```python
from build123d import *

# Parameters (mm, degrees)
IZIM1_W               = 153
IZIM1_H               = 12.405405405
KES_EKSTR_ZYON1_DEPTH = 21
KES_EKSTR_ZYON2_START = -21
KES_EKSTR_ZYON2_DEPTH = 21


with BuildPart() as part:
    # Çizim1 → Döndür1 (revolve)
    with BuildSketch(Plane(origin=(0, 0, 0), x_dir=(-1, 0, 0), z_dir=(0, 0, -1)), mode=Mode.PRIVATE) as d_nd_r1_sk:
        with Locations((-76.5, 6.202702703)):
            Rectangle(IZIM1_W, IZIM1_H)
    revolve(d_nd_r1_sk.sketch.rotate(Axis((153, 0, 0), (-1, 0, 0)), 270), axis=Axis((153, 0, 0), (-1, 0, 0)))

    # Çizim2 → Kes-Ekstrüzyon1 (cut)
    with BuildSketch(Plane(origin=(153, 0, 0), x_dir=(0, 0, -1), z_dir=(1, 0, 0))):
        with BuildLine():
            Line((5.478492651, -2.446654506), (11.327153725, -5.058623505))
            ThreePointArc((11.327153725, -5.058623505), (0.113988201, -12.404881699), (-11.232281693, -5.26592169))
            Line((-11.232281693, -5.26592169), (-5.432606832, -2.546916373))
            ThreePointArc((-5.432606832, -2.546916373), (-0.055131548, 5.999746704), (5.478492651, -2.446654506))
        make_face()
    extrude(amount=-KES_EKSTR_ZYON1_DEPTH, mode=Mode.SUBTRACT)

    # Çizim3 → Kes-Ekstrüzyon2 (cut)
    with BuildSketch(Plane.ZY.offset(KES_EKSTR_ZYON2_START)):
        with BuildLine():
            ThreePointArc((2.25, -5.562148865), (0, 6), (-2.25, -5.562148865))
            ThreePointArc((-2.25, -5.562148865), (0, -6), (2.25, -5.562148865))
        make_face()
    extrude(amount=KES_EKSTR_ZYON2_DEPTH, mode=Mode.SUBTRACT)


solid = part.part
```
Design review of the part built by this model. Coordinates are the model's own, in mm. A direction names the side the tool comes from. Give positions to 0.01 mm unless a question says otherwise; leave off trailing zeros. Order: outer loops, then holes, each group sorted by start corner. A loop starts at its lowest first (then second) coordinate and runs counter-clockwise, first axis right, second up. Notation, with made-up numbers: M -25.5,12.5 L 23.5,12.5 A24 ccw 23.5,44.5 Z; hole C 50,-28 d5. An arc over 180 degrees is marked long. One line per question, with ' | ' between items. Start each with the question number.
Q1. For L1, parallel to Z at x = 145.75, y = 0; L2, parallel to Y at x = 146, z = 0; L3, parallel to X at y = -2.75, z = 2, list the stretches that pass through material, from the lowest coordinate up. Write a range as [from, to].
Q2. We need section B-B (y = 0). Write out the cut boundary in (x, z), plus the area to 3 significant figures.
Q3. Machinability: for faces 1 (the face through (142.647, -3.925, 8.373)), 2 (the face through (143, 6, 0)), 3 (the face through (153, 6, -3)), 4 (the face through (21, 0, 0)), which of the approach directions +Z, -Z, +X, -X, +Y, -Y give a long, thin tool a straight path to every point of the face, cutting with its end or side? Answer none if there is none.
Q4. The part is to be moulded in two halves that separate along Z. For faces 5 (the face through (0, -3, 6)), 6 (the face through (75.4, 12.3, -1.6)), 7 (the face through (142.647, -3.734, -8.362)), say which applies: +Z half, -Z half, draft (parallel to the pull), parting line (faces both ways), or undercut.
Q5. For pin 1 Ø4 at (x, y) = (96, 7.5) entering from -Z; pin 2 Ø6 at (x, z) = (22.5, 8.5) entering from +Y; pin 3 Ø4 at (x, z) = (97, 5.5) entering from +Y; pin 4 Ø13 at (y, z) = (-3, 1) entering from -X, all flat-tipped, find the tip position at first contact; note any pin that passes through.
Q6. We need section D-D (x = 13). Write out the cut boundary in (y, z), plus the area to 3 significant figures.
Q7. We need section C-C (x = 37.5). Write out the cut boundary in (y, z), plus the area to 3 significant figures.
Q8. We need section A-A (z = 0). Write out the cut boundary in (x, y).
Returned:
1) L1: [-12.41, -6], [6, 12.41] | L2: [6, 12.41] | L3: [21, 132]
2) outline: M 0,-12.41 L 153,-12.41 L 153,-6 L 132,-6 L 132,6 L 153,6 L 153,12.41 L 0,12.41 L 0,6 L 21,6 L 21,-6 L 0,-6 Z | area: 3,290 mm2
3) face 1: +X, -Y | face 2: +X | face 3: +Z, -Z, +X, +Y, -Y | face 4: -X
4) face 5: draft | face 6: parting line | face 7: undercut
5) pin 1: z = -11.12 | pin 2: y = 11.12 | pin 3: y = 11.9 | pin 4: x = 0
6) outline: C 0,0 d24.81; hole C 0,0 d12 | area: 370 mm2
7) outline: C 0,0 d24.81 | area: 483 mm2
8) outline: M 0,-12.41 L 132,-12.41 L 132,6 L 153,6 L 153,12.41 L 0,12.41 L 0,6 L 21,6 L 21,-6 L 0,-6 Z
